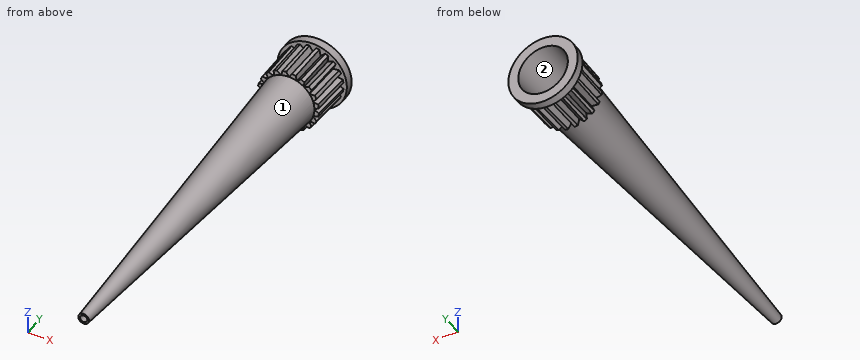
from build123d import *

# Parameters (mm, degrees)
IZIM2_R               = 3
KES_EKSTR_ZYON1_DEPTH = 49
KES_EKSTR_ZYON1_TAPER = 3
KES_EKSTR_ZYON4_DEPTH = 5
SCALE1_SCALE          = 0.880952381


with BuildPart() as part:
    # Çizim1 → Döndür1 (revolve)
    with BuildSketch(Plane.XY):
        Polygon((0, 0), (0, 49), (4.2, 49), (4.2, 48), (3.8, 48), (3.7, 43), (3.15, 43), (0.65, 0), align=None)
    revolve(axis=Axis((0, 0, 0), (0, 1, 0)))

    # Çizim2 → Kes-Ekstrüzyon1 (cut)
    with BuildSketch(Plane(origin=(0, 49, 0), x_dir=(1, 0, 0), z_dir=(0, 1, 0))):
        Circle(IZIM2_R)
    extrude(amount=-KES_EKSTR_ZYON1_DEPTH, taper=KES_EKSTR_ZYON1_TAPER, mode=Mode.SUBTRACT)

    # Çizim3 → Kes-Ekstrüzyon4 (cut)
    with BuildSketch(Plane.XZ.offset(-43)):
        Polygon((0.08224501, 3.1), (-0.41775499, 3.966025404), (0.58224501, 3.966025404), align=None)
        Polygon((0.815256969, 3.918905719), (1.766313485, 3.609888725), (1.02316866, 2.940758119), align=None)
        Polygon((1.973360244, 3.493070587), (2.782377238, 2.905285335), (1.868831781, 2.498548692), align=None)
        Polygon((2.943191617, 2.730203716), (3.53097687, 1.921186722), (2.536454974, 1.816658258), align=None)
        Polygon((3.629817237, 1.704979831), (3.938834232, 0.753923315), (2.960686631, 0.961835006), align=None)
        Polygon((3.966025404, 0.51775499), (3.966025404, -0.48224501), (3.1, 0.01775499), align=None)
        Polygon((3.918905719, -0.715256969), (3.609888725, -1.666313485), (2.940758119, -0.92316866), align=None)
        Polygon((3.493070587, -1.873360244), (2.905285335, -2.682377238), (2.498548692, -1.768831781), align=None)
        Polygon((2.730203716, -2.843191617), (1.921186722, -3.43097687), (1.816658258, -2.436454974), align=None)
        Polygon((1.704979831, -3.529817237), (0.753923315, -3.838834232), (0.961835006, -2.860686631), align=None)
        Polygon((0.51775499, -3.866025404), (-0.48224501, -3.866025404), (0.01775499, -3), align=None)
        Polygon((-0.715256969, -3.818905719), (-1.666313485, -3.509888725), (-0.92316866, -2.840758119), align=None)
        Polygon((-1.873360244, -3.393070587), (-2.682377238, -2.805285335), (-1.768831781, -2.398548692), align=None)
        Polygon((-2.843191617, -2.630203716), (-3.43097687, -1.821186722), (-2.436454974, -1.716658258), align=None)
        Polygon((-3.529817237, -1.604979831), (-3.838834232, -0.653923315), (-2.860686631, -0.861835006), align=None)
        Polygon((-3.866025404, -0.41775499), (-3.866025404, 0.58224501), (-3, 0.08224501), align=None)
        Polygon((-3.818905719, 0.815256969), (-3.509888725, 1.766313485), (-2.840758119, 1.02316866), align=None)
        Polygon((-3.393070587, 1.973360244), (-2.805285335, 2.782377238), (-2.398548692, 1.868831781), align=None)
        Polygon((-2.630203716, 2.943191617), (-1.821186722, 3.53097687), (-1.716658258, 2.536454974), align=None)
        Polygon((-1.604979831, 3.629817237), (-0.653923315, 3.938834232), (-0.861835006, 2.960686631), align=None)
    extrude(amount=-KES_EKSTR_ZYON4_DEPTH, mode=Mode.SUBTRACT)


with BuildPart() as part_1:
    # Scale1: scaled about (0.02225364, 34.813303108, 0.02225364)
    add(part.part.scale(SCALE1_SCALE).moved(Location((0.002649243, 4.144440846, 0.002649243))))


solid = part_1.part
Work out the finished part from the listing and answer in its coordinate system (mm). Face numbers are marked on the shaded views. Round coordinates to 2 decimals unless told otherwise and drop trailing zeros. Loops run counter-clockwise (first coordinate to the right, second up) from the corner with the lowest first, then second, coordinate; pieces in that order, holes last. Notation, with made-up numbers: M -8.5,89.5 L 27.5,89.5 A19 cw 27.5,106.5 Z; hole C -7.75,67 d6. An arc over 180 degrees is marked long. One line per question, with ' | ' between items. Start each with the question number.
(1) A cutting plane is placed at A-A on y = 13. Write down the section's boundary in (x, z), plus the area to 3 significant figures.
(2) Find the intervals of material crossed by line 1 (X direction, y = 43, z = -1.75); line 2 (Y direction, x = 1.5, z = 2.75); line 3 (X direction, y = 30, z = 0.5), in increasing order.
(3) For a pull along X with two mould halves and no side action, classify the marked faces 1 and 2 as released by +X, released by -X, zero draft, split by the parting line, or undercut.
(4) A flat-ended cylindrical pin translates along its axis: pin 1 Ø4 at (x, y) = (1.5, 14) entering from +Z. Find the tip coordinate at first contact, or state that the pin passes through.
(5) A cutting plane is placed at B-B on y = 8.5. Write down the section's boundary in (x, z), plus the area to 3 significant figures.
Geometry check:
1) outline: C 0,0 d2.17; hole C 0,0 d1.69 | area: 1.47 mm²
2) line 1: x = -2.25 to -1.66, 1.67 to 2.29 | line 2: y = 42.03 to 47.31 | line 3: x = -2.01 to -1.66, 1.67 to 2.02
3) face 1: split by the parting line | face 2: undercut
4) pin 1: stops at z = 1.23
5) outline: C 0,0 d1.65; hole C 0,0 d1.22 | area: 0.978 mm²
